Read the model definition and answer for the solid it produces. Units are mm, in the model's axes. A direction names the side the tool comes from. Give positions to 0.01 mm unless a question says otherwise; leave off trailing zeros. Order: outer loops, then holes, each group sorted by start corner. A loop starts at its lowest first (then second) coordinate and runs counter-clockwise, first axis right, second up. Notation, with made-up numbers: (40.25, 1.25) - (77.25, 1.25) arc R19 cw to (77.25, 25.25) - close; hole circle Ø5 at (45.5, -8). An arc over 180 degrees is marked (long way). Return JSON: item names as keys, results as strings.
Autodesk Inventor part; units mm, degrees
ref_plane "D2X1_XY" through (5.5, 16, 0) normal (0, 0, 1) x (1, 0, 0)
ref_plane "D2X1_YZ" through (5.5, 16, 0) normal (1, 0, 0) x (0, 1, 0)
ref_plane "D2X1_ZX" through (5.5, 16, 0) normal (0, 1, 0) x (0, 0, 1)
sketch "Skizze_1" plane through (0, 0, 0) normal (0, 0, 1) x (1, 0, 0)
  line L0 (5.5, 0) -> (-5.5, 0)
  line L1 (-5.5, 15) -> (-5.5, 7)
  line L2 (-5.5, 7) -> (5.5, 7)
  line L3 (5.5, 7) -> (5.5, 15)
  arc A0 (5.5, 15) -> (4.5, 16) centre (4.5, 15) ccw
  line L4 (4.5, 16) -> (-4.5, 16)
  arc A1 (-4.5, 16) -> (-5.5, 15) centre (-4.5, 15) ccw
revolve "Revolution1" add sketch "Skizze_1" angle 360 about axis through (5.5, 0, 0) along (1, 0, 0)
sketch "Sketch_4" plane through (0, 0, 0) normal (1, 0, 0) x (0, 0, -1)
  line L0 (-21, 0.6) -> (-21, -0.6)
  line L1 (-21, -0.6) -> (13, -0.6)
  line L2 (13, -0.6) -> (13, 0.6)
  line L3 (13, 0.6) -> (-21, 0.6)
extrude "Extrusion1" cut sketch "Sketch_4" along normal mid plane 22
sketch "Sketch_6" plane through (0, 0, 13) normal (0, 0, 1) x (1, 0, 0)
  line L0 (0, 0) -> (0, 21)
  line L1 (0, 21) -> (4, 21)
  line L2 (4, 21) -> (4, 4.6)
  line L3 (4, 4.6) -> (2.25, 4.6)
  line L4 (2.25, 4.6) -> (2.25, 0)
  line L5 (2.25, 0) -> (0, 0)
  line L6 (0, 0) -> (0, 21)
revolve "Revolution2" cut sketch "Sketch_6" angle 360 about axis through (0, 0, 13) along (0, -1, 0)
sketch "Sketch_2" plane through (0, 11.5, 0) normal (0, 1, 0) x (1, 0, 0)
  line L0 (5.5, 0) -> (-5.5, 0)
  line L1 (-5.5, 0) -> (-5.5, 2)
  line L2 (-5.5, 2) -> (-5.121, 1.621)
  line L3 (-5.121, 1.621) -> (5.121, 1.621)
  line L4 (5.121, 1.621) -> (5.5, 2)
  line L5 (5.5, 2) -> (5.5, 0)
  line L6 (5.5, 0) -> (-5.5, 0)
revolve "Revolution3" cut sketch "Sketch_2" angle 360 about axis through (5.5, 11.5, 0) along (1, 0, 0)
thread "Thread1"
sketch "Sketch_3" plane through (0, -11.5, 0) normal (0, 1, 0) x (1, 0, 0)
  line L0 (5.5, 0) -> (-5.5, 0)
  line L1 (-5.5, 0) -> (-5.5, 2)
  line L2 (-5.5, 2) -> (-5.121, 1.621)
  line L3 (-5.121, 1.621) -> (5.121, 1.621)
  line L4 (5.121, 1.621) -> (5.5, 2)
  line L5 (5.5, 2) -> (5.5, 0)
  line L6 (5.5, 0) -> (-5.5, 0)
revolve "Revolution4" cut sketch "Sketch_3" angle 360 about axis through (5.5, -11.5, 0) along (1, 0, 0)
thread "Thread2"
sketch "Sketch_1" plane through (0, 0, 0) normal (1, 0, 0) x (0, 0, -1)
  line L0 (-13, -9.5555) -> (-13, -0.6)
  line L1 (-13, -0.6) -> (-10.5, -0.6)
  line L2 (-10.5, -0.6) -> (-11, -1.1)
  line L3 (-11, -1.1) -> (-11, -11.8471)
  line L4 (-11, -11.8471) -> (-13, -9.5555)
  line L5 (-13, -9.5555) -> (-13, -0.6)
revolve "Revolution5" cut sketch "Sketch_1" angle 360 about axis through (0, -9.5555, 13) along (0, -1, 0)
ref_plane "D2X1_XY" through (5.5, 16, 0) normal (0, 0, 1) x (1, 0, 0)
ref_plane "D2X1_YZ" through (5.5, 16, 0) normal (1, 0, 0) x (0, 1, 0)
ref_plane "D2X1_ZX" through (5.5, 16, 0) normal (0, 1, 0) x (0, 0, 1)
ref_plane "D2X2_XY" through (5.5, -16, 0) normal (0, 0, 1) x (1, 0, 0)
ref_plane "D2X2_YZ" through (5.5, -16, 0) normal (1, 0, 0) x (0, 1, 0)
ref_plane "D2X2_ZX" through (5.5, -16, 0) normal (0, 1, 0) x (0, 0, 1)
ref_plane "schraubenkopf_XY" through (0, 4.6, 13) normal (0, 1, 0) x (1, 0, 0)
ref_plane "schraubenkopf_YZ" through (0, 4.6, 13) normal (1, 0, 0) x (0, 0, -1)
ref_plane "schraubenkopf_ZX" through (0, 4.6, 13) normal (0, 0, -1) x (0, 1, 0)
properties part number "62311400GA_1"
Q1. A cutting plane is placed at A-A (x = 0). Write down the section's boundary in (y, z), and give its area (3 significant figures).
Values:
{"outline": "(-11.62, 11) arc R16 ccw (long way) to (13.23, 9) - (4.6, 9) - (4.6, 10.75) - (0.6, 10.75) - (0.6, 6.97) arc R7 cw to (0.6, -6.97) - (0.6, -13) - (-0.6, -13) - (-0.6, -6.97) arc R7 cw to (-0.6, 6.97) - (-0.6, 10.5) - (-1.1, 11) - close; (-5.57, 15) - (-1.1, 15) - (-0.6, 15.5) - (-0.6, 15.99) arc R16 ccw to start; (0.6, 15.25) - (4.6, 15.25) - (4.6, 15.32) arc R16 ccw to (0.6, 15.99) - close; hole circle Ø3.24 at (-11.5, 0); hole circle Ø3.24 at (11.5, 0)", "area": "530 mm²"}
Q2. A cutting plane is placed at B-B (z = 13). Give the number of separate pieces and of enclosed holes in the cut face, and give its area (3 significant figures).
Values:
{"separate pieces": "4", "enclosed holes": "0", "area": "99.5 mm²"}
Q3. Consider L1, parallel to Y at x = 0.5, z = 0; L2, parallel to Z at x = -1.5, y = 3; L3, parallel to Y at x = -4.25, z = 1. Determine where each line is inside the solid, lowest interval first.
Values:
{"L1": "y = -16 to -13.12, -9.88 to -7, 7 to 9.88, 13.12 to 16", "L2": "z = -15.72 to -6.32, 6.32 to 11.32, 14.68 to 15.72", "L3": "y = -15.97 to -12.78, -10.22 to -6.93, 6.93 to 10.22, 12.78 to 15.97"}
Q4. Given pin 1 (3 mm diameter, centred on x = 2, z = -10.5, fed in from -Y); pin 2 (2 mm diameter, centred on x = -1.5, z = -8.5, fed in from +Y); pin 3 (1 mm diameter, centred on x = -1, z = -3, fed in from -Y), each flat-ended and moving along its own axis, determine where each tip first touches the part or whether it passes through.
Values:
{"pin 1": "stops at y = -13.23", "pin 2": "stops at y = 14.13", "pin 3": "stops at y = -15.8"}
Q5. For faces 1 (the cylindrical face through (-0.29, 2.57, 15.23)), 2 (the flat face through (0, 0.6, 10)), 3 (the cylindrical face through (0, -7, 0)), determine the directions among +Z, -Z, +X, -X, +Y, -Y from which every point of the face is accessible in a straight line to the end or side of a thin tool.
Values:
{"face 1": "+Y", "face 2": "+Z, +X, -X", "face 3": "+X, -X"}
Q6. Determine the mould class of faces 4 (the flat face through (0, 4.6, 10)), 5 (the flat face through (0, 0, -13)), 6 (the flat face through (-1.3, -0.6, 10.5)) for opening direction Z: released by +Z, released by -Z, zero draft, split by the parting line, or undercut.
Values:
{"face 4": "undercut", "face 5": "released by +Z", "face 6": "zero draft"}
